Check sheet for the modelled part. Datum: model origin and axes. Units: mm. A direction names the side the tool comes from. Round coordinates to 2 decimals unless told otherwise and drop trailing zeros. Write each loop counter-clockwise with the first axis right and the second up, starting at its lowest first coordinate (ties: lowest second). Pieces come first, ordered by that corner, then holes. Notation, with made-up numbers: (-16, -23.5) - (-9, -23.5) arc R18 ccw to (-9, 7.5) - close; hole circle Ø1 at (87, 86.5). An arc over 180 degrees is marked (long way). Use one line per item in the form item = value. Start each with the question number.
1) Section check A-A (y = 8.25). Record the boundary of the cut face in (x, z), then the cut area to 4 significant figures.
2) Section check B-B (x = 8.05). Record the boundary of the cut face in (y, z), then the cut area to 3 significant figures.
3) Gauge pin test, flat ends, axial feed: P1, Ø4, axis at x = 42.5, z = 51, coming from the -Y side; P2, Ø0.8, axis at x = 18.5, z = 70, coming from the +Y side; P3, Ø3, axis at y = 5.5, z = 11.5, coming from the -X side; P4, Ø1.5, axis at x = 26.5, z = 25.5, coming from the +Y side. Record the tip position at first contact, or that the pin passes through.
4) Set-up check for faces 4 (the face through (-8, 2, 52)), 5 (the face through (8, 12, 79)): record each of +Z, -Z, +X, -X, +Y, -Y from which the full face is reachable in a straight line by a thin tool's end or side.
5) Section check C-C (z = 21). Record the boundary of the cut face in (x, y).
6) Draft check along Z on faces 1 (the face through (81, 6, -2)), 2 (the face through (74, 0, 31)), 3 (the face through (165, 7, 28)). Enter one of: +Z half, -Z half, draft (parallel to the pull), parting line (faces both ways), or undercut.
7) Scan lines: probe 1 along X at (y, z) = (6, 51.7); probe 2 along X at (y, z) = (5.75, 12); probe 3 along Z at (x, y) = (69, 11). Record each from-to range of solid material in increasing order.
8) Section check D-D (z = 51.7). Record the boundary of the cut face in (x, y).
from build123d import *

# Parameters (mm, degrees)
SKETCH_1_W          = 165
SKETCH_1_H          = 56
EXTRUDE_1_DEPTH     = 2
SKETCH_3_W          = 169
SKETCH_3_H          = 60
SKETCH_3_W_2        = 165
SKETCH_3_H_2        = 56
EXTRUDE_2_DEPTH     = 12
SKETCH_4_R          = 10.05
EXTRUDE_3_DEPTH     = 2
SKETCH_5_R          = 12.05
SKETCH_5_R_2        = 10.05
EXTRUDE_4_DEPTH     = 12
SKETCH_6_W          = 46.432971474
SKETCH_6_H          = 8
CUT_EXTRUDE_1_DEPTH = 9
SKETCH_7_R          = 6.3
EXTRUDE_5_DEPTH     = 2
SKETCH_8_R          = 8.3
SKETCH_8_R_2        = 6.3
EXTRUDE_6_DEPTH     = 12


with BuildPart() as part:
    # Sketch 1 → Extrude 1 (new body)
    with BuildSketch(Plane(origin=(0, 0, 0), x_dir=(1, 0, 0), z_dir=(0, 1, 0))):
        with Locations((82.5, -28)):
            Rectangle(SKETCH_1_W, SKETCH_1_H)
    extrude(amount=EXTRUDE_1_DEPTH)

    # Sketch 3 → Extrude 2 (add)
    with BuildSketch(Plane.XZ):
        with Locations((82.5, 28)):
            Rectangle(SKETCH_3_W, SKETCH_3_H)
        with Locations((82.5, 28)):
            Rectangle(SKETCH_3_W_2, SKETCH_3_H_2, mode=Mode.SUBTRACT)
    extrude(amount=-EXTRUDE_2_DEPTH)



with BuildPart() as body_2:
    # Sketch 4 → Extrude 3 (new body)
    with BuildSketch(Plane.XZ):
        with Locations(Location((8.05, 68.05, 0), (0, 0, 270))):
            Circle(SKETCH_4_R)
    extrude(amount=-EXTRUDE_3_DEPTH)


with BuildPart() as part_1:
    add(part.part)

    add(body_2.part)  # Extrude 4 merges body 2
    # Sketch 5 → Extrude 4 (add)
    with BuildSketch(Plane.XZ):
        with Locations((8.05, 68.05)):
            Circle(SKETCH_5_R)
        with Locations(Location((8.05, 68.05, 0), (0, 0, 270))):
            Circle(SKETCH_5_R_2, mode=Mode.SUBTRACT)
    extrude(amount=-EXTRUDE_4_DEPTH)

    # Sketch 6 → Cut-Extrude 1 (cut)
    with BuildSketch(Plane(origin=(0, 12, 0), x_dir=(1, 0, 0), z_dir=(0, 1, 0))):
        with Locations((8.05, -68.05)):
            Rectangle(SKETCH_6_W, SKETCH_6_H)
    extrude(amount=-CUT_EXTRUDE_1_DEPTH, mode=Mode.SUBTRACT)



with BuildPart() as body_2_2:
    # Sketch 7 → Extrude 5 (new body)
    with BuildSketch(Plane.XZ):
        with Locations(Location((-8.3, 51.7, 0), (0, 0, 270))):
            Circle(SKETCH_7_R)
    extrude(amount=-EXTRUDE_5_DEPTH)


with BuildPart() as part_2:
    add(part_1.part)

    add(body_2_2.part)  # Extrude 6 merges body 2 2
    # Sketch 8 → Extrude 6 (add)
    with BuildSketch(Plane.XZ):
        with Locations((-8.3, 51.7)):
            Circle(SKETCH_8_R)
        with Locations(Location((-8.3, 51.7, 0), (0, 0, 270))):
            Circle(SKETCH_8_R_2, mode=Mode.SUBTRACT)
    extrude(amount=-EXTRUDE_6_DEPTH)


solid = part_2.part
Results are:
q1.outline = (-3.32, 64.05) arc R12.05 ccw to (1.4, 58) - (-2, 58) - (-2, 57.1) arc R8.3 ccw (long way) to (-2, 46.3) - (-2, -2) - (167, -2) - (167, 58) - (14.7, 58) arc R12.05 ccw to (19.42, 64.05) - (17.27, 64.05) arc R10.05 cw to (-1.17, 64.05) - close; (-3.32, 72.05) - (-1.17, 72.05) arc R10.05 cw to (17.27, 72.05) - (19.42, 72.05) arc R12.05 ccw to start; hole circle Ø12.6 at (-8.3, 51.7); hole (0, 0) - (165, 0) - (165, 56) - (0, 56) - close
q1.area = 1,065 mm²
q2.outline = (0, -2) - (12, -2) - (12, 0) - (2, 0) - (2, 56) - (12, 56) - (12, 58) - (2, 58) - (2, 78.1) - (12, 78.1) - (12, 80.1) - (0, 80.1) - close
q2.area = 224 mm²
q3.P1 = 0
q3.P2 = 3
q3.P3 = -2
q3.P4 = 2
q4.face_4 = +Y
q4.face_5 = +Z, -Z, +X, -X, +Y
q5.outline = (-2, 0) - (167, 0) - (167, 12) - (165, 12) - (165, 2) - (0, 2) - (0, 12) - (-2, 12) - close
q6.face_1 = -Z half
q6.face_2 = draft
q6.face_3 = undercut
q7.probe_1 = -16.6 to -14.6, -2 to 0, 165 to 167
q7.probe_2 = -2 to 0, 165 to 167
q7.probe_3 = -2 to 0, 56 to 58
q8.outline = (-16.6, 0) - (167, 0) - (167, 12) - (165, 12) - (165, 2) - (0, 2) - (0, 12) - (-2, 12) - (-2, 2) - (-14.6, 2) - (-14.6, 12) - (-16.6, 12) - close
